For this review, take the finished solid that the model builds, in its own axes (mm). Give positions to 0.01 mm unless a question says otherwise; leave off trailing zeros. Write each loop counter-clockwise with the first axis right and the second up, starting at its lowest first coordinate (ties: lowest second). Pieces come first, ordered by that corner, then holes. Notation, with made-up numbers: M 82,61.5 L 91,61.5 A22 ccw 91,88.5 Z; hole C -16.5,-28 d4. An arc over 180 degrees is marked long. Use one line per item in the form item = value. Start each with the question number.
Q1. Consider section B-B on x = -7.5. Write out the cut boundary in (y, z).
Q2. Mouldability with a two-part tool opening along Y and no side actions: class faces 1 (the cylindrical face through (18.802, 27.014, -0.493)), 2 (the cylindrical face through (-24.204, -18.559, -0.493)), 3 (the flat face through (1, 31, 0)), 4 (the flat face through (41.09, 23.98, -0.49)) as released by +Y, released by -Y, zero draft, split by the parting line, or undercut.
Q3. Consider section A-A on z = -0.25. Write out the cut boundary in (x, y).
Q4. Clearance check with a flat-ended pin moving along its axis: pin 1 Ø5 at (x, y) = (39, 8) entering from +Z. State where the tip first meets the part, or that it passes through.
Q5. Consider section C-C on y = 35. Write out the cut boundary in (x, z), and give its area (3 significant figures).
Q6. For probe 1 along Y at (x, z) = (0, -0.2); probe 2 along Y at (x, z) = (24, -0.7); probe 3 along Y at (x, z) = (26, -0.15), list the stretches that pass through material, from the lowest coordinate up. Write a range as [from, to].
Q7. Consider section D-D on x = -22. Write out the cut boundary in (y, z).
```python
from build123d import *

# Parameters (mm, degrees)
SKETCH1_R           = 30.5
SKETCH1_R_2         = 6.55
SKETCH1_R_3         = 4.05
BOSS_EXTRUDE1_DEPTH = 1


with BuildPart() as part:
    # Sketch1 → Boss-Extrude1 (new body)
    with BuildSketch(Plane.XY):
        with BuildLine():
            Line((0, 45), (24.742465391, 42.399462096))
            ThreePointArc((24.742465391, 42.399462096), (30.023792252, 40.529246167), (33.880428677, 36.465199352))
            Line((33.880428677, 36.465199352), (48.5, 11.143359036))
            Line((48.5, 11.143359036), (48.5, 3.143359036))
            Line((48.5, 3.143359036), (35.471224905, -32.652906339))
            ThreePointArc((35.471224905, -32.652906339), (31.908364772, -37.741197937), (26.278691588, -40.366357655))
            Line((26.278691588, -40.366357655), (0, -45))
            Line((0, -45), (-26.278691588, -40.366357655))
            ThreePointArc((-26.278691588, -40.366357655), (-31.908364772, -37.741197937), (-35.471224905, -32.652906339))
            Line((-35.471224905, -32.652906339), (-48.5, 3.143359036))
            Line((-48.5, 3.143359036), (-48.5, 11.143359036))
            Line((-48.5, 11.143359036), (-33.880428677, 36.465199352))
            ThreePointArc((-33.880428677, 36.465199352), (-30.023792252, 40.529246167), (-24.742465391, 42.399462096))
            Line((-24.742465391, 42.399462096), (0, 45))
        make_face()
        Circle(SKETCH1_R, mode=Mode.SUBTRACT)
        with Locations((24, 31)):
            Circle(SKETCH1_R_2, mode=Mode.SUBTRACT)
        with Locations(Location((-24, 31, 0), (0, 0, 180))):
            Circle(SKETCH1_R_2, mode=Mode.SUBTRACT)
        with Locations((-25, -30)):
            Circle(SKETCH1_R_2, mode=Mode.SUBTRACT)
        with Locations(Location((25, -30, 0), (0, 0, 180))):
            Circle(SKETCH1_R_2, mode=Mode.SUBTRACT)
        with Locations((39, 8)):
            Circle(SKETCH1_R_3, mode=Mode.SUBTRACT)
        with Locations(Location((-39, 8, 0), (0, 0, 180))):
            Circle(SKETCH1_R_3, mode=Mode.SUBTRACT)
    extrude(amount=-BOSS_EXTRUDE1_DEPTH)


solid = part.part
```
Working result:
q1.outline = M -43.68,-1 L -29.56,-1 L -29.56,0 L -43.68,0 Z; M 29.56,-1 L 44.21,-1 L 44.21,0 L 29.56,0 Z
q2.face_1 = undercut
q2.face_2 = undercut
q2.face_3 = zero draft
q2.face_4 = released by +Y
q3.outline = M -48.5,3.14 L -35.47,-32.65 A12 ccw -26.28,-40.37 L 0,-45 L 26.28,-40.37 A12 ccw 35.47,-32.65 L 48.5,3.14 L 48.5,11.14 L 33.88,36.47 A12 ccw 24.74,42.4 L 0,45 L -24.74,42.4 A12 ccw -33.88,36.47 L -48.5,11.14 Z; hole C -39,8 d8.1; hole C -25,-30 d13.1; hole C -24,31 d13.1; hole C 0,0 d61; hole C 24,31 d13.1; hole C 25,-30 d13.1; hole C 39,8 d8.1
q4.pin_1 = through
q5.outline = M -34.73,-1 L -29.19,-1 L -29.19,0 L -34.73,0 Z; M -18.81,-1 L 18.81,-1 L 18.81,0 L -18.81,0 Z; M 29.19,-1 L 34.73,-1 L 34.73,0 L 29.19,0 Z
q5.area = 48.7 mm²
q6.probe_1 = [-45, -30.5], [30.5, 45]
q6.probe_2 = [-40.77, -36.47], [-23.53, -18.82], [18.82, 24.45], [37.55, 42.48]
q6.probe_3 = [-40.42, -36.47], [-23.53, -15.95], [15.95, 24.76], [37.24, 42.2]
q7.outline = M -41.12,-1 L -35.82,-1 L -35.82,0 L -41.12,0 Z; M -24.18,-1 L -21.12,-1 L -21.12,0 L -24.18,0 Z; M 21.12,-1 L 24.76,-1 L 24.76,0 L 21.12,0 Z; M 37.24,-1 L 42.69,-1 L 42.69,0 L 37.24,0 Z
